from build123d import *

# Parameters (mm, degrees)
F0_R     = 40
F1_DEPTH = 400
F6_R     = 20


with BuildPart() as f1:
    # F0 (on Top) → F1 (new body)
    with BuildSketch(Plane.XY):
        Circle(F0_R)
    extrude(amount=-F1_DEPTH)

    # F2 (on Front) → F3 (revolve, cut)
    with BuildSketch(Plane.XZ):
        Polygon((-40, 0), (-40, -10), (-30, 0), align=None)
    revolve(axis=Axis((0, 0, -3.875099), (0, 0, -1)), mode=Mode.SUBTRACT)

    # F4 (on Front) → F5 (revolve)
    with BuildSketch(Plane.XZ):
        Polygon((-30, 0), (0, 0), (0, 116.126455), align=None)
    revolve(axis=Axis((0, 0, 58.063228), (0, 0, 1)))

    # F6
    f6_edges = [f1.edges().sort_by_distance(p)[0] for p in [
        (30, 0, 0),
    ]]
    fillet(f6_edges, radius=F6_R)

    # F7 (on Front) → F8 (revolve)
    with BuildSketch(Plane.XZ):
        Polygon((0, -400), (-40, -400), (0, -600), align=None)
    revolve(axis=Axis((0, 0, -500), (0, 0, -1)))


solid = f1.part
For this review, take the finished solid that the model builds, in its own axes (mm). Give positions to 0.01 mm unless a question says otherwise; leave off trailing zeros. Loops run counter-clockwise (first coordinate to the right, second up) from the corner with the lowest first, then second, coordinate; pieces in that order, holes last. Notation, with made-up numbers: M -10,-13.75 L 7,-13.75 A18 ccw 7,-7.75 Z; hole C -19.75,-20.5 d10. An arc over 180 degrees is marked long. Answer as a JSON object with one key per item and string values. Group by question number.
Q1. Insertion check: P1, Ø12, axis at x = -17.5, z = -366.5, coming from the +Y side; P2, Ø3, axis at x = -5.5, z = -122.5, coming from the -Y side; P3, Ø12, axis at x = 18.5, z = -49, coming from the -Y side. Each pin has a flat end and moves straight along its axis. Give the tip position at first contact, or say it passes through.
Q2. Add section B-B on z = -408. Give the boundary of the cut face in (x, y).
Q3. Add section A-A on z = -293. Give the boundary of the cut face in (x, y).
Q4. For probe 1 along X at (y, z) = (1, -271); probe 2 along Y at (x, z) = (-20, -323.5); probe 3 along X at (y, z) = (25, -361), list the stretches that pass through material, from the lowest coordinate up. Write a range as [from, to].
Checked values:
{
 "1": {"P1": "y = 38.31", "P2": "y = -39.8", "P3": "y = -38"},
 "2": {"outline": "C 0,0 d76.8"},
 "3": {"outline": "C 0,0 d80"},
 "4": {"probe 1": "[-39.99, 39.99]", "probe 2": "[-34.64, 34.64]", "probe 3": "[-31.22, 31.22]"}
}
